Part model, mm, in its own coordinate system. Face numbers are marked on the shaded views. A direction names the side the tool comes from. Give positions to 0.01 mm unless a question says otherwise; leave off trailing zeros. Write each loop counter-clockwise with the first axis right and the second up, starting at its lowest first coordinate (ties: lowest second). Pieces come first, ordered by that corner, then holes.
Autodesk Inventor part; units mm, degrees
ref_plane "YZ Plane" through (0, 0, 0) normal (1, 0, 0) x (0, 1, 0)
ref_plane "XZ Plane" through (0, 0, 0) normal (0, 1, 0) x (-1, 0, 0)
ref_plane "XY Plane" through (0, 0, 0) normal (0, 0, 1) x (1, 0, 0)
sketch "Sketch1" plane through (0, 0, 0) normal (0, 0, 1) x (1, 0, 0)
  arc A0 (-33, 0) -> (33, 0) centre (0, 0) ccw
  arc A1 (-27, 0) -> (27, 0) centre (0, 0) ccw
  line L0 (-33, 0) -> (-27, 0)
  line L1 (27, 0) -> (33, 0)
  dimension "d0" = 66
  dimension "d1" = 54
extrude "Extrusion1" add sketch "Sketch1" along normal blind 10
sketch "Sketch2" plane through (-33, 0, 0) normal (0, 1, 0) x (1, 0, 0)
  line L0 (6, 0) -> (6, -10)
  line L1 (6, 0) -> (-9, 0)
  line L2 (-9, 0) -> (-9, -10)
  line L3 (-9, -10) -> (6, -10)
  line L4 (6, -10) -> (6, 0)
  line L5 (66, 0) -> (60, 0)
  line L6 (60, 0) -> (75, 0)
  line L7 (75, 0) -> (75, -10)
  line L8 (75, -10) -> (60, -10)
  line L9 (60, -10) -> (60, 0)
  point P0 (33, 0)
  dimension "d4" = 15
extrude "Extrusion2" add sketch "Sketch2" against normal blind 5
sketch "Sketch3" plane through (-27, 0, 10) normal (0, 1, 0) x (1, 0, 0)
  circle A0 centre (-9, 5) radius 1.65
  circle A1 centre (63, 5) radius 1.65
  line L0 (0, 10) -> (-15, 10)
  line L1 (-15, 10) -> (-15, 0)
  line L2 (69, 10) -> (54, 10)
  line L3 (69, 0) -> (69, 10)
  point P0 (27, 10)
  dimension "d7" = 5
  dimension "d8" = 6
  dimension "d9" = 5
  dimension "d10" = 6
  dimension "d11" = 3.3
extrude "Extrusion3" cut sketch "Sketch3" against normal blind 5
fillet "Fillet1" radius 2 4 edges at (-27, 0, 5) (-32.619, -5, 5) (32.619, -5, 5) (27, 0, 5)
properties part number "22010B_Tube End Support_V2" material "ABS Plastic"
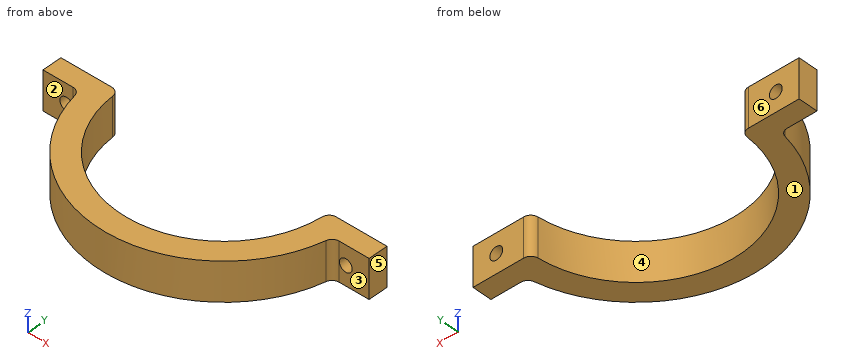
1) Saw through at C-C, the plane y = -22. Write the cut outline in (x, z).
Answers follow:
outline: (-24.6, 0) - (-15.65, 0) - (-15.65, 10) - (-24.6, 10) - close; (15.65, 0) - (24.6, 0) - (24.6, 10) - (15.65, 10) - close
2) Pin check, flat tips, straight feed: pin 1 Ø4 at (x, z) = (38.5, 6) entering from -Y; pin 2 Ø5 at (y, z) = (-10, 2) entering from +X; pin 3 Ø1 at (y, z) = (-28, 7.5) entering from +X. Stop position of each tip, or through.
Answers follow:
pin 1: stops at y = -5
pin 2: stops at x = 32.14
pin 3: stops at x = 18.24
3) Saw through at D-D, the plane x = 0. Write the cut outline in (y, z).
Answers follow:
outline: (-33, 0) - (-27, 0) - (-27, 10) - (-33, 10) - close
4) Wall check: L1, parallel to X at y = -2, z = 9; L2, parallel to Z at x = 36, y = -2.2; L3, parallel to X at y = -4.5, z = 1.5. Give the ranges that are in metal, low to high.
Answers follow:
L1: x = -42 to -26.93, 26.93 to 42
L2: z = 0 to 3.35, 6.65 to 10
L3: x = -42 to -26.62, 26.62 to 42
5) Two-plate mould, pull along X, no slides. Class the marked faces 4, 5 and 6: +X half, -X half, draft (parallel to the pull), parting line (faces both ways), or undercut.
Answers follow:
face 4: undercut
face 5: +X half
face 6: draft
6) 3-axis set-ups, long thin cutter, end or side, ignore diameter. For the marked faces 1, 2 and 3: which of +Z, -Z, +X, -X, +Y, -Y reach the whole face in a straight line?
Answers follow:
face 1: -Z, +X, -X, +Y, -Y
face 2: +Z, -Z, -X, -Y
face 3: +Z, -Z, +X, -Y
7) Saw through at B-B, the plane x = -36. Write the cut outline in (y, z).
Answers follow:
outline: (-5, 0) - (0, 0) - (0, 3.35) - (-5, 3.35) - close; (-5, 6.65) - (0, 6.65) - (0, 10) - (-5, 10) - close
